Answer from the drawing. Dimensions are ordinates in mm from the lowest x, y and z of the part. A direction names the side the tool comes from. Give positions to 0.01 mm unless a question says otherwise; leave off trailing zeros. Loops run counter-clockwise (first coordinate to the right, second up) from the corner with the lowest first, then second, coordinate; pieces in that order, holes last. Notation, with made-up numbers: M -39,24.5 L -12,24.5 A6 ccw -12,32.5 Z; hole C 19.25,54.5 d7. An arc over 180 degrees is marked long. Use a Markdown table: item, result.
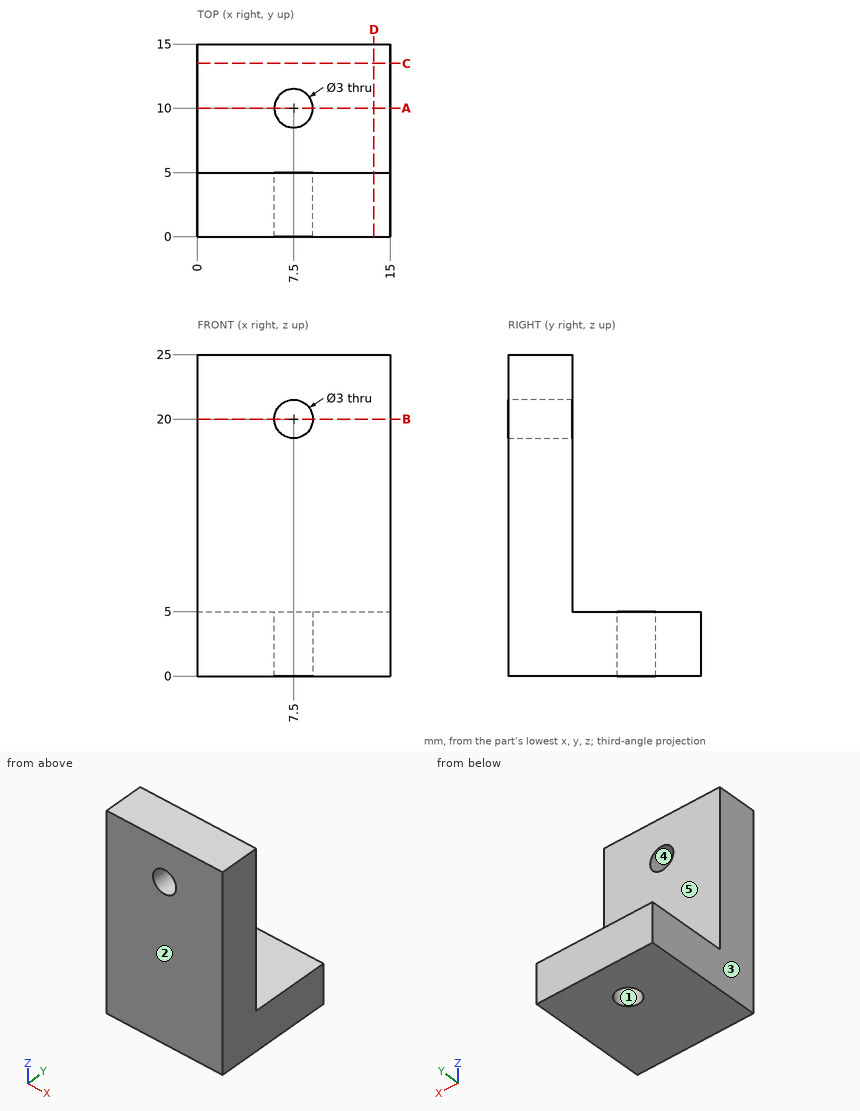
(1) Which of the six approach directions +Z, -Z, +X, -X, +Y, -Y give full straight-line access (tool end or side, diameter ignored) to the marked faces 4 and 5?
Entries:
| item | result |
|---|---|
| face 4 | +Y, -Y |
| face 5 | +Z, +X, -X, +Y |
(2) Given P1, Ø5, axis at x = 7.5, y = 10, coming from the +Z side; P2, Ø7.5, axis at x = 7, z = 14, coming from the +Y side, each flat-ended and moving along its own axis, determine where each tip first touches the part or whether it passes through.
Entries:
| item | result |
|---|---|
| P1 | stops at z = 5 |
| P2 | stops at y = 5 |
(3) Consider probe 1 along Y at (x, z) = (7.5, 2.55); probe 2 along X at (y, z) = (3.7, 20); probe 3 along Y at (x, z) = (14.25, 10.25). Determine where each line is inside the solid, lowest interval first. Write a range as [from, to].
Entries:
| item | result |
|---|---|
| probe 1 | y = [0, 8.5], [11.5, 15] |
| probe 2 | x = [0, 6], [9, 15] |
| probe 3 | y = [0, 5] |
(4) A cutting plane is placed at A-A (y = 10). Write down the section's boundary in (x, z), and give its area (3 significant figures).
Entries:
| item | result |
|---|---|
| outline | M 0,0 L 6,0 L 6,5 L 0,5 Z; M 9,0 L 15,0 L 15,5 L 9,5 Z |
| area | 60.0 mm² |
(5) The mould has two halves that part along Y. Classify the marked faces 1, 2 and 3: released by +Y, released by -Y, zero draft, split by the parting line, or undercut.
Entries:
| item | result |
|---|---|
| face 1 | undercut |
| face 2 | released by -Y |
| face 3 | zero draft |
(6) A cutting plane is placed at D-D (x = 13.75). Write down the section's boundary in (y, z).
Entries:
| item | result |
|---|---|
| outline | M 0,0 L 15,0 L 15,5 L 5,5 L 5,25 L 0,25 Z |
(7) A cutting plane is placed at C-C (y = 13.5). Write down the section's boundary in (x, z), and give its area (3 significant figures).
Entries:
| item | result |
|---|---|
| outline | M 0,0 L 15,0 L 15,5 L 0,5 Z |
| area | 75.0 mm² |
